Build history of the part. All positions in model axes, mm. A direction names the side the tool comes from. Give positions to 0.01 mm unless a question says otherwise; leave off trailing zeros. Order: outer loops, then holes, each group sorted by start corner. A loop starts at its lowest first (then second) coordinate and runs counter-clockwise, first axis right, second up. Notation, with made-up numbers: (-12, -21.5) -> (29, -21.5) arc R8 ccw to (29, -12.5) -> close; hole circle Ø5 at (-34, -2.5). An arc over 180 degrees is marked (long way). One line per question, with ' | ' between items. Start each with the question number.
(1) Cut at A-A (x = 42.5). Give the cut face in (y, z).
(2) Pull direction Y, two halves, no side cores. Call faces 4 (the face through (79, 24, 7)), 5 (the face through (39, 35, 4)), 6 (the face through (39, 0, 4)): +Y half, -Y half, draft (parallel to the pull), parting line (faces both ways), or undercut.
(3) Cut at C-C (z = 3). Give the cut face in (x, y).
(4) Which spindle directions (+Z, -Z, +X, -X, +Y, -Y) get a long thin tool onto all of the face, cutting with end or side? Do faces 1 (the face through (79, 11, 7)), 2 (the face through (0, 17, 4)), 3 (the face through (78, 17.3, 5.7)). Say none if no direction does.
(5) Drill centre lines: L1, parallel to X at y = 32.5, z = 3.25; L2, parallel to Y at x = 77.5, z = 5.5; L3, parallel to Y at x = 21, z = 7. Where is each one in solid material? Low to high. Write a range as from..to.
(6) Cut at B-B (y = 8). Give the cut face in (x, z).
(7) Pin check, flat tip, straight feed: pin 1 Ø0.5 at (x, y) = (38.5, 1.5) entering from +Z. Stop position of the tip, or through.
(8) Cut at D-D (x = 13). Give the cut face in (y, z), then the cut area to 3 significant figures.
from build123d import *

# Parameters (mm, degrees)
BOX009_W             = 41
BOX009_H             = 1
BOX009_DEPTH         = 2
BOX008_W             = 41
BOX008_H             = 1
BOX008_DEPTH         = 2
CYLINDER004_R        = 1.5
CYLINDER004_DEPTH    = 10
CYLINDER003_R        = 1.5
CYLINDER003_DEPTH    = 10
CYLINDER002_R        = 1.5
CYLINDER002_DEPTH    = 10
CYLINDER001_R        = 1.5
CYLINDER001_DEPTH    = 10
BOX005_W             = 3
BOX005_H             = 25
BOX005_DEPTH         = 10
BOX004_W             = 2
BOX004_H             = 16
BOX004_DEPTH         = 9
BOX003_W             = 2
BOX003_H             = 13
BOX003_DEPTH         = 5
BOX002_W             = 2
BOX002_H             = 25
BOX002_DEPTH         = 9
CYLINDER_R           = 3
CYLINDER_DEPTH       = 2
CYLINDER_PITCH_ANGLE = 90
BOX001_W             = 69
BOX001_H             = 25
BOX001_DEPTH         = 13
BOX_W                = 80
BOX_H                = 35
BOX_DEPTH            = 8.5


with BuildPart() as box009:
    # Box009 → Box009 (new body)
    with BuildSketch(Plane(origin=(19.5, 1, 6.5), x_dir=(1, 0, 0), z_dir=(0, 0, 1))):
        with Locations((20.5, 0.5)):
            Rectangle(BOX009_W, BOX009_H)
    extrude(amount=BOX009_DEPTH)


with BuildPart() as box008:
    # Box008 → Box008 (new body)
    with BuildSketch(Plane(origin=(19.5, 33, 6.5), x_dir=(1, 0, 0), z_dir=(0, 0, 1))):
        with Locations((20.5, 0.5)):
            Rectangle(BOX008_W, BOX008_H)
    extrude(amount=BOX008_DEPTH)


with BuildPart() as cylinder004:
    # Cylinder004 → Cylinder004 (new body)
    with BuildSketch(Plane(origin=(2.5, 32.5, 0), x_dir=(1, 0, 0), z_dir=(0, 0, 1))):
        Circle(CYLINDER004_R)
    extrude(amount=CYLINDER004_DEPTH)


with BuildPart() as cylinder003:
    # Cylinder003 → Cylinder003 (new body)
    with BuildSketch(Plane(origin=(77.5, 32.5, 0), x_dir=(1, 0, 0), z_dir=(0, 0, 1))):
        Circle(CYLINDER003_R)
    extrude(amount=CYLINDER003_DEPTH)


with BuildPart() as cylinder002:
    # Cylinder002 → Cylinder002 (new body)
    with BuildSketch(Plane(origin=(77.5, 2.5, 0), x_dir=(1, 0, 0), z_dir=(0, 0, 1))):
        Circle(CYLINDER002_R)
    extrude(amount=CYLINDER002_DEPTH)


with BuildPart() as cylinder001:
    # Cylinder001 → Cylinder001 (new body)
    with BuildSketch(Plane(origin=(2.5, 2.5, 0), x_dir=(1, 0, 0), z_dir=(0, 0, 1))):
        Circle(CYLINDER001_R)
    extrude(amount=CYLINDER001_DEPTH)


with BuildPart() as box005:
    # Box005 → Box005 (new body)
    with BuildSketch(Plane(origin=(2, 5, 2), x_dir=(1, 0, 0), z_dir=(0, 0, 1))):
        with Locations((1.5, 12.5)):
            Rectangle(BOX005_W, BOX005_H)
    extrude(amount=BOX005_DEPTH)


with BuildPart() as box004:
    # Box004 → Box004 (new body)
    with BuildSketch(Plane(origin=(74, 9.5, 4), x_dir=(1, 0, 0), z_dir=(0, 0, 1))):
        with Locations((1, 8)):
            Rectangle(BOX004_W, BOX004_H)
    extrude(amount=BOX004_DEPTH)


with BuildPart() as u:
    # Box003 → Box003 (new body)
    with BuildSketch(Plane(origin=(78, 11, 6), x_dir=(1, 0, 0), z_dir=(0, 0, 1))):
        with Locations((1, 6.5)):
            Rectangle(BOX003_W, BOX003_H)
    extrude(amount=BOX003_DEPTH)


with BuildPart() as box002:
    # Box002 → Box002 (new body)
    with BuildSketch(Plane(origin=(76, 5, 4), x_dir=(1, 0, 0), z_dir=(0, 0, 1))):
        with Locations((1, 12.5)):
            Rectangle(BOX002_W, BOX002_H)
    extrude(amount=BOX002_DEPTH)


with BuildPart() as cylinder:
    # Cylinder → Cylinder (new body)
    with BuildSketch(Plane.XY):
        Circle(CYLINDER_R)
    extrude(amount=CYLINDER_DEPTH)


with BuildPart() as cylinder_1:
    # Cylinder pitch: moved
    add(cylinder.part.rotate(Axis((0, 0, 0), (0, 1, 0)), CYLINDER_PITCH_ANGLE))


with BuildPart() as cylinder_2:
    # Cylinder placement: moved
    add(cylinder_1.part.moved(Location((0, 17.5, 8.5))))


with BuildPart() as box001:
    # Box001 → Box001 (new body)
    with BuildSketch(Plane(origin=(5, 5, 2), x_dir=(1, 0, 0), z_dir=(0, 0, 1))):
        with Locations((34.5, 12.5)):
            Rectangle(BOX001_W, BOX001_H)
    extrude(amount=BOX001_DEPTH)


with BuildPart() as cut011:
    # Box → Box (new body)
    with BuildSketch(Plane.XY):
        with Locations((40, 17.5)):
            Rectangle(BOX_W, BOX_H)
    extrude(amount=BOX_DEPTH)

    # Cut: cut Box001
    add(box001.part, mode=Mode.SUBTRACT)

    # Cut001: cut Cylinder
    add(cylinder_2.part, mode=Mode.SUBTRACT)

    # Cut002: cut Box002
    add(box002.part, mode=Mode.SUBTRACT)

    add(u.part, mode=Mode.SUBTRACT)

    # Cut004: cut Box004
    add(box004.part, mode=Mode.SUBTRACT)

    # Cut005: cut Box005
    add(box005.part, mode=Mode.SUBTRACT)

    # Cut006: cut Cylinder001
    add(cylinder001.part, mode=Mode.SUBTRACT)

    # Cut007: cut Cylinder002
    add(cylinder002.part, mode=Mode.SUBTRACT)

    # Cut008: cut Cylinder003
    add(cylinder003.part, mode=Mode.SUBTRACT)

    # Cut009: cut Cylinder004
    add(cylinder004.part, mode=Mode.SUBTRACT)

    # Cut010: cut Box008
    add(box008.part, mode=Mode.SUBTRACT)

    # Cut011: cut Box009
    add(box009.part, mode=Mode.SUBTRACT)


solid = cut011.part
Result set:
1) outline: (0, 0) -> (35, 0) -> (35, 8.5) -> (34, 8.5) -> (34, 6.5) -> (33, 6.5) -> (33, 8.5) -> (30, 8.5) -> (30, 2) -> (5, 2) -> (5, 8.5) -> (2, 8.5) -> (2, 6.5) -> (1, 6.5) -> (1, 8.5) -> (0, 8.5) -> close
2) face 4: undercut | face 5: +Y half | face 6: -Y half
3) outline: (0, 0) -> (80, 0) -> (80, 35) -> (0, 35) -> close; hole circle Ø3 at (2.5, 2.5); hole circle Ø3 at (2.5, 32.5); hole (2, 5) -> (74, 5) -> (74, 30) -> (2, 30) -> close; hole circle Ø3 at (77.5, 2.5); hole circle Ø3 at (77.5, 32.5)
4) face 1: +Z, +X | face 2: +Z, -Z, -X, +Y, -Y | face 3: +Z
5) L1: x = 0..1, 4..76, 79..80 | L2: y = 0..1, 4..5, 30..31, 34..35 | L3: y = 0..1, 2..5, 30..33, 34..35
6) outline: (0, 0) -> (80, 0) -> (80, 8.5) -> (78, 8.5) -> (78, 4) -> (76, 4) -> (76, 8.5) -> (74, 8.5) -> (74, 2) -> (2, 2) -> (2, 8.5) -> (0, 8.5) -> close
7) pin 1: stops at z = 6.5
8) outline: (0, 0) -> (35, 0) -> (35, 8.5) -> (30, 8.5) -> (30, 2) -> (5, 2) -> (5, 8.5) -> (0, 8.5) -> close | area: 135 mm2
